from build123d import *

# Parameters (mm, degrees)
F0_R           = 0.8
F0_W           = 13
F0_H           = 12
F1_DEPTH       = 5
F2_W           = 13
F2_H           = 6
F3_DEPTH       = 0.5
F5_D           = 2
F5_DEPTH       = 20
F5_CBORE_D     = 4
F5_CBORE_DEPTH = 1.5
F5_TIP         = 0.600860619
F6_R           = 10
F7_R           = 3
F8_T1_DEPTH    = 4.1430571099
F8_T3_DEPTH    = 9.217139142
F8_T5_DEPTH    = 16
F8_T7_DEPTH    = 9.0537269763
F8_T9_DEPTH    = 9.217139142
F8_T12_ANGLE   = 90
F8_T14_ANGLE   = 105.2904097565
F8_T16_ANGLE   = 90
F8_T18_ANGLE   = 15.2904100724
F8_T20_ANGLE   = 15.2904100724
F8_T22_ANGLE   = 105.2904094573


# Not quite as in the source:
# - a fillet or chamfer that OpenCascade refuses, or shapes differently, is made with other operations: its cross-section is extruded or revolved along the edge and cut away or added


with BuildPart() as f1:
    # F0 (on Top) → F1 (new body)
    with BuildSketch(Plane.XY):
        Polygon((-18, -7.25), (18, -7.25), (18, 7.25), (4.9295582736, 7.25), (-4.9295582736, 7.25), (-18, 7.25), align=None)
        with Locations((-9, 0)):
            Circle(F0_R, mode=Mode.SUBTRACT)
        Rectangle(F0_W, F0_H, mode=Mode.SUBTRACT)
        with Locations((9, 0)):
            Circle(F0_R, mode=Mode.SUBTRACT)
        with BuildLine():
            Line((4.9295582736, 7.25), (18, 7.25))
            ThreePointArc((18, 7.25), (17.6073787038, 9), (16.5047771245, 10.4145392323))
            Line((16.5047771245, 10.4145392323), (4.9295582736, 7.25))
        make_face()
        with BuildLine():
            ThreePointArc((-16.5047771245, 10.4145392323), (-17.6073787038, 9), (-18, 7.25))
            Line((-18, 7.25), (-4.9295582736, 7.25))
            Line((-4.9295582736, 7.25), (-16.5047771245, 10.4145392323))
        make_face()
    extrude(amount=F1_DEPTH)

    # F2 (on face) → F3 (join)
    with BuildSketch(Plane(origin=(0, 0, 0), x_dir=(1, 0, 0), z_dir=(0, 0, -1))):
        Rectangle(F2_W, F2_H)
    extrude(amount=-F3_DEPTH)

    # F5
    with Locations(Plane.XY.offset(5)):
        with Locations((-15, 0), (15, 0)):
            CounterBoreHole(F5_D / 2, F5_CBORE_D / 2, F5_CBORE_DEPTH, depth=F5_DEPTH)
            with Locations((0, 0, -(F5_DEPTH + F5_TIP / 2))):  # 118° drill point
                Cone(0, F5_D / 2, F5_TIP, mode=Mode.SUBTRACT)

    # F6
    f6_edges = [f1.edges().sort_by_distance(p)[0] for p in [
        (-18, -7.25, 2.5),
        (18, -7.25, 2.5),
    ]]
    fillet(f6_edges, radius=F6_R)

    # F7
    f7_edges = [f1.edges().sort_by_distance(p)[0] for p in [
        (-16.504777, 10.414539, 2.5),
        (16.504777, 10.414539, 2.5),
        (-4.929558, 7.25, 2.5),
        (4.929558, 7.25, 2.5),
    ]]
    fillet(f7_edges, radius=F7_R)

    # F8: fillet of radius 1 on 12 edges, made by hand

    # F8_s2 → F8_t1 (cut)
    with BuildSketch(Plane.XZ.offset(-6.8930571099)):
        with BuildLine():
            ThreePointArc((-18, 4), (-17.7071067812, 4.7071067812), (-17, 5))
            Line((-17, 5), (-18, 5))
            Line((-18, 5), (-18, 4))
        make_face()
        with BuildLine():
            ThreePointArc((18, 4), (17.7071067812, 4.7071067812), (17, 5))
            Line((17, 5), (18, 5))
            Line((18, 5), (18, 4))
        make_face()
    extrude(amount=F8_T1_DEPTH, mode=Mode.SUBTRACT)

    # F8_s4 → F8_t3 (cut)
    with BuildSketch(Plane(origin=(-6.8194085753, 1.8643523078, 0), x_dir=(0, 0, 1), z_dir=(-0.9646015709, 0.2637116027, 0))):
        with BuildLine():
            ThreePointArc((4, 5.6933796762), (4.7071067812, 5.4004864574), (5, 4.6933796762))
            Line((5, 4.6933796762), (5, 5.6933796762))
            Line((5, 5.6933796762), (4, 5.6933796762))
        make_face()
    extrude(amount=F8_T3_DEPTH, mode=Mode.SUBTRACT)

    # F8_s6 → F8_t5 (cut)
    with BuildSketch(Plane.YZ.offset(-8)):
        with BuildLine():
            ThreePointArc((-7.25, 4), (-6.9571067812, 4.7071067812), (-6.25, 5))
            Line((-6.25, 5), (-7.25, 5))
            Line((-7.25, 5), (-7.25, 4))
        make_face()
    extrude(amount=F8_T5_DEPTH, mode=Mode.SUBTRACT)

    # F8_s8 → F8_t7 (cut)
    with BuildSketch(Plane.YZ.offset(-4.5268634881)):
        with BuildLine():
            ThreePointArc((7.25, 4), (6.9571067812, 4.7071067812), (6.25, 5))
            Line((6.25, 5), (7.25, 5))
            Line((7.25, 5), (7.25, 4))
        make_face()
    extrude(amount=F8_T7_DEPTH, mode=Mode.SUBTRACT)

    # F8_s10 → F8_t9 (cut)
    with BuildSketch(Plane(origin=(15.7102754711, 4.2950188431, 0), x_dir=(0, 0, 1), z_dir=(-0.9646015709, -0.2637116027, 0))):
        with BuildLine():
            ThreePointArc((4, 5.6933796762), (4.7071067812, 5.4004864574), (5, 4.6933796762))
            Line((5, 4.6933796762), (5, 5.6933796762))
            Line((5, 5.6933796762), (4, 5.6933796762))
        make_face()
    extrude(amount=F8_T9_DEPTH, mode=Mode.SUBTRACT)

    # F8_s11 → F8_t12 (revolve, cut)
    with BuildSketch(Plane.YZ.offset(8)):
        with BuildLine():
            ThreePointArc((-7.25, 4), (-6.9571067812, 4.7071067812), (-6.25, 5))
            Line((-6.25, 5), (-7.25, 5))
            Line((-7.25, 5), (-7.25, 4))
        make_face()
    revolve(axis=Axis((8, 2.75, 5), (0, 0, 1)), revolution_arc=F8_T12_ANGLE, mode=Mode.SUBTRACT)

    # F8_s13 → F8_t14 (revolve, cut)
    with BuildSketch(Plane.XZ.offset(-6.8930571003)):
        with BuildLine():
            ThreePointArc((-18.0000000058, 4), (-17.707106787, 4.7071067812), (-17.0000000058, 5))
            Line((-17.0000000058, 5), (-18, 5))
            Line((-18, 5), (-18.0000000058, 4))
        make_face()
    revolve(axis=Axis((-14.9999999954, 6.8930571003, 5), (0, 0, -1)), revolution_arc=F8_T14_ANGLE, mode=Mode.SUBTRACT)

    # F8_s15 → F8_t16 (revolve, cut)
    with BuildSketch(Plane.YZ.offset(-8)):
        with BuildLine():
            ThreePointArc((-7.25, 4), (-6.9571067812, 4.7071067812), (-6.25, 5))
            Line((-6.25, 5), (-7.25, 5))
            Line((-7.25, 5), (-7.25, 4))
        make_face()
    revolve(axis=Axis((-8, 2.75, 5), (0, 0, -1)), revolution_arc=F8_T16_ANGLE, mode=Mode.SUBTRACT)

    # F8_s17 → F8_t18 (revolve, cut)
    with BuildSketch(Plane(origin=(-6.8194085753, 1.8643523078, 0), x_dir=(0, 0, 1), z_dir=(-0.9646015709, 0.2637116027, 0))):
        with BuildLine():
            ThreePointArc((4, 5.6933796762), (4.7071067812, 5.4004864574), (5, 4.6933796762))
            Line((5, 4.6933796762), (5, 5.6933796762))
            Line((5, 5.6933796762), (4, 5.6933796762))
        make_face()
    revolve(axis=Axis((-4.5268634881, 10.25, 5), (0, 0, 1)), revolution_arc=F8_T18_ANGLE, mode=Mode.SUBTRACT)

    # F8_s19 → F8_t20 (revolve, cut)
    with BuildSketch(Plane(origin=(6.8194085753, 1.8643523078, 0), x_dir=(0, 0, 1), z_dir=(0.9646015709, 0.2637116027, 0))):
        with BuildLine():
            ThreePointArc((4, -5.6933796762), (4.7071067812, -5.4004864574), (5, -4.6933796762))
            Line((5, -4.6933796762), (5, -5.6933796762))
            Line((5, -5.6933796762), (4, -5.6933796762))
        make_face()
    revolve(axis=Axis((4.5268634881, 10.25, 5), (0, 0, -1)), revolution_arc=F8_T20_ANGLE, mode=Mode.SUBTRACT)

    # F8_s21 → F8_t22 (revolve, cut)
    with BuildSketch(Plane.XZ.offset(-6.8930570951)):
        with BuildLine():
            ThreePointArc((18.0000000063, 4), (17.7071067875, 4.7071067812), (17.0000000063, 5))
            Line((17.0000000063, 5), (18, 5))
            Line((18, 5), (18.0000000063, 4))
        make_face()
    revolve(axis=Axis((14.999999986, 6.8930570951, 5), (0, 0, 1)), revolution_arc=F8_T22_ANGLE, mode=Mode.SUBTRACT)


solid = f1.part
Can you work these out from the model? Positions are in its coordinate system, mm. A direction names the side the tool comes from. Coordinates: 2 decimals unless noted, no trailing zeros. Write each loop counter-clockwise with the first axis right and the second up, starting at its lowest first coordinate (ties: lowest second). Pieces come first, ordered by that corner, then holes. Notation, with made-up numbers: (32.5, 89) -> (40.5, 89) arc R26 ccw to (40.5, 118) -> close; hole circle Ø1 at (-31, 15). An arc over 180 degrees is marked (long way). Write each question's results on one line, items separated by ' | '. Start each with the question number.
Item 1: Thinking about a two-plate mould opening in Y: for faces 6 (the cylindrical face through (14.99, -4.4, 2.03)), 7 (the flat face through (0, 0, 0.5)), 8 (the flat face through (9.83, 8.59, 1.97)), which applies, released by +Y, released by -Y, zero draft, split by the parting line, or undercut?
Item 2: Please list where these lines run through material, in increasing order: probe 1 along Y at (x, z) = (-2.5, 0.4); probe 2 along Y at (x, z) = (1, 2.1); probe 3 along Z at (x, y) = (4.5, 0.5).
Item 3: If we section it at B-B, the plane z = 1.1: Count the separate pieces of the cut face and the enclosed holes in it, and give its area (3 significant figures).
Item 4: If we section it at A-A, the plane x = 3: Write out the boundary of the cut face in (y, z), and give its area (3 significant figures).
Item 5: I'm going to push flat-ended pins straight in: P1, Ø5, axis at x = 2.5, y = 1, coming from the +Z side; P2, Ø3.5, axis at x = 15, y = 0, coming from the +Z side; P3, Ø4, axis at x = -3, y = -5, coming from the -Z side; P4, Ø1, axis at y = -4, z = 2, coming from the +X side. Where does each tip first touch, or does it pass through?
Item 6: On a 3-axis mill with a long thin cutter (end or side, diameter ignored), from which of +Z, -Z, +X, -X, +Y, -Y can I reach the whole of each face in a straight line? I mean faces 1 (the flat face through (0, 7.25, 2)), 2 (the cylindrical face through (-14.99, -4.4, 2.03)), 3 (the cylindrical face through (-13.092, 0.601, 4.261)), 4 (the cylindrical face through (-9.78, 8.28, 4.7)), 5 (the flat face through (0, 6, 2)). Say none if no direction works.
Answer block:
1) face 6: released by -Y | face 7: undercut | face 8: released by +Y
2) probe 1: -7.25 to -6, -3 to 3, 6 to 7.25 | probe 2: -7.25 to -6, 6 to 7.25 | probe 3: 0 to 0.5
3) separate pieces: 1 | enclosed holes: 5 | area: 352 mm²
4) outline: (-7.25, 0) -> (-6, 0) -> (-6, 5) -> (-6.25, 5) arc R1 ccw to (-7.25, 4) -> close; (-3, 0) -> (3, 0) -> (3, 0.5) -> (-3, 0.5) -> close; (6, 0) -> (7.25, 0) -> (7.25, 4) arc R1 ccw to (6.25, 5) -> (6, 5) -> close | area: 15.1 mm²
5) P1: z = 0.5 | P2: z = 3.5 | P3: z = 0 | P4: x = 15.81
6) face 1: +Z, -Z, +Y | face 2: +Z, -Z, -X, -Y | face 3: +Z | face 4: +Z, +Y | face 5: +Z, -Z
